from build123d import *

# Parameters (mm, degrees)
F1_DEPTH = 2


with BuildPart() as f1:
    # F0 (on Top) → F1 (new body)
    with BuildSketch(Plane.XY):
        with BuildLine():
            Line((-167, 135.5), (-167, 137.5))
            Line((-167, 137.5), (-169, 137.5))
            Line((-169, 137.5), (-172, 137.5))
            Line((-172, 137.5), (-172, 0))
            Line((-172, 0), (-170, 0))
            Line((-170, 0), (-170, 2))
            ThreePointArc((-170, 2), (-169.853553, 2.353553), (-169.5, 2.5))
            Line((-169.5, 2.5), (-167, 2.5))
            Line((-167, 2.5), (-167, 3.5))
            Line((-167, 3.5), (-167, 5.5))
            Line((-167, 5.5), (-167, 6.5))
            Line((-167, 6.5), (-169.5, 6.5))
            ThreePointArc((-169.5, 6.5), (-169.853553, 6.646447), (-170, 7))
            Line((-170, 7), (-170, 15))
            ThreePointArc((-170, 15), (-169.853553, 15.353553), (-169.5, 15.5))
            Line((-169.5, 15.5), (-167, 15.5))
            Line((-167, 15.5), (-167, 16.5))
            Line((-167, 16.5), (-167, 18.5))
            Line((-167, 18.5), (-167, 19.5))
            Line((-167, 19.5), (-169.5, 19.5))
            ThreePointArc((-169.5, 19.5), (-169.853553, 19.646447), (-170, 20))
            Line((-170, 20), (-170, 28))
            ThreePointArc((-170, 28), (-169.853553, 28.353553), (-169.5, 28.5))
            Line((-169.5, 28.5), (-167, 28.5))
            Line((-167, 28.5), (-167, 29.5))
            Line((-167, 29.5), (-167, 31.5))
            Line((-167, 31.5), (-167, 32.5))
            Line((-167, 32.5), (-169.5, 32.5))
            ThreePointArc((-169.5, 32.5), (-169.853553, 32.646447), (-170, 33))
            Line((-170, 33), (-170, 41))
            ThreePointArc((-170, 41), (-169.853553, 41.353553), (-169.5, 41.5))
            Line((-169.5, 41.5), (-167, 41.5))
            Line((-167, 41.5), (-167, 42.5))
            Line((-167, 42.5), (-167, 44.5))
            Line((-167, 44.5), (-167, 45.5))
            Line((-167, 45.5), (-169.5, 45.5))
            ThreePointArc((-169.5, 45.5), (-169.853553, 45.646447), (-170, 46))
            Line((-170, 46), (-170, 54))
            ThreePointArc((-170, 54), (-169.853553, 54.353553), (-169.5, 54.5))
            Line((-169.5, 54.5), (-167, 54.5))
            Line((-167, 54.5), (-167, 55.5))
            Line((-167, 55.5), (-167, 57.5))
            Line((-167, 57.5), (-167, 58.5))
            Line((-167, 58.5), (-169.5, 58.5))
            ThreePointArc((-169.5, 58.5), (-169.853553, 58.646447), (-170, 59))
            Line((-170, 59), (-170, 67))
            ThreePointArc((-170, 67), (-169.853553, 67.353553), (-169.5, 67.5))
            Line((-169.5, 67.5), (-167, 67.5))
            Line((-167, 67.5), (-167, 68.5))
            Line((-167, 68.5), (-167, 70.5))
            Line((-167, 70.5), (-167, 71.5))
            Line((-167, 71.5), (-169.5, 71.5))
            ThreePointArc((-169.5, 71.5), (-169.853553, 71.646447), (-170, 72))
            Line((-170, 72), (-170, 80))
            ThreePointArc((-170, 80), (-169.853553, 80.353553), (-169.5, 80.5))
            Line((-169.5, 80.5), (-167, 80.5))
            Line((-167, 80.5), (-167, 81.5))
            Line((-167, 81.5), (-167, 83.5))
            Line((-167, 83.5), (-167, 84.5))
            Line((-167, 84.5), (-169.5, 84.5))
            ThreePointArc((-169.5, 84.5), (-169.853553, 84.646447), (-170, 85))
            Line((-170, 85), (-170, 93))
            ThreePointArc((-170, 93), (-169.853553, 93.353553), (-169.5, 93.5))
            Line((-169.5, 93.5), (-167, 93.5))
            Line((-167, 93.5), (-167, 94.5))
            Line((-167, 94.5), (-167, 96.5))
            Line((-167, 96.5), (-167, 97.5))
            Line((-167, 97.5), (-169.5, 97.5))
            ThreePointArc((-169.5, 97.5), (-169.853553, 97.646447), (-170, 98))
            Line((-170, 98), (-170, 106))
            ThreePointArc((-170, 106), (-169.853553, 106.353553), (-169.5, 106.5))
            Line((-169.5, 106.5), (-167, 106.5))
            Line((-167, 106.5), (-167, 107.5))
            Line((-167, 107.5), (-167, 109.5))
            Line((-167, 109.5), (-167, 110.5))
            Line((-167, 110.5), (-169.5, 110.5))
            ThreePointArc((-169.5, 110.5), (-169.853553, 110.646447), (-170, 111))
            Line((-170, 111), (-170, 119))
            ThreePointArc((-170, 119), (-169.853553, 119.353553), (-169.5, 119.5))
            Line((-169.5, 119.5), (-167, 119.5))
            Line((-167, 119.5), (-167, 120.5))
            Line((-167, 120.5), (-167, 122.5))
            Line((-167, 122.5), (-167, 123.5))
            Line((-167, 123.5), (-169.5, 123.5))
            ThreePointArc((-169.5, 123.5), (-169.853553, 123.646447), (-170, 124))
            Line((-170, 124), (-170, 132))
            ThreePointArc((-170, 132), (-169.853553, 132.353553), (-169.5, 132.5))
            Line((-169.5, 132.5), (-167, 132.5))
            Line((-167, 132.5), (-167, 133.5))
            Line((-167, 133.5), (-167, 135.5))
        make_face()
        Polygon((-167, 5.5), (-167, 3.5), (-165.5, 3.5), (-165.5, 3), (-165, 3.5), (-165, 5.5), (-165.5, 6), (-165.5, 5.5), align=None)
        Polygon((-167, 18.5), (-167, 16.5), (-165.5, 16.5), (-165.5, 16), (-165, 16.5), (-165, 18.5), (-165.5, 19), (-165.5, 18.5), align=None)
        Polygon((-167, 31.5), (-167, 29.5), (-165.5, 29.5), (-165.5, 29), (-165, 29.5), (-165, 31.5), (-165.5, 32), (-165.5, 31.5), align=None)
        Polygon((-167, 44.5), (-167, 42.5), (-165.5, 42.5), (-165.5, 42), (-165, 42.5), (-165, 44.5), (-165.5, 45), (-165.5, 44.5), align=None)
        Polygon((-167, 57.5), (-167, 55.5), (-165.5, 55.5), (-165.5, 55), (-165, 55.5), (-165, 57.5), (-165.5, 58), (-165.5, 57.5), align=None)
        Polygon((-165.5, 70.5), (-167, 70.5), (-167, 68.5), (-165.5, 68.5), (-165.5, 68), (-165, 68.5), (-165, 70.5), (-165.5, 71), align=None)
        Polygon((-165.5, 83.5), (-167, 83.5), (-167, 81.5), (-165.5, 81.5), (-165.5, 81), (-165, 81.5), (-165, 83.5), (-165.5, 84), align=None)
        Polygon((-165.5, 96.5), (-167, 96.5), (-167, 94.5), (-165.5, 94.5), (-165.5, 94), (-165, 94.5), (-165, 96.5), (-165.5, 97), align=None)
        Polygon((-165.5, 109.5), (-167, 109.5), (-167, 107.5), (-165.5, 107.5), (-165.5, 107), (-165, 107.5), (-165, 109.5), (-165.5, 110), align=None)
        Polygon((-165.5, 122.5), (-167, 122.5), (-167, 120.5), (-165.5, 120.5), (-165.5, 120), (-165, 120.5), (-165, 122.5), (-165.5, 123), align=None)
        Polygon((-165.5, 135.5), (-167, 135.5), (-167, 133.5), (-165.5, 133.5), (-165.5, 133), (-165, 133.5), (-165, 135.5), (-165.5, 136), align=None)
        with BuildLine():
            Line((-169, 137.5), (-167, 137.5))
            Line((-167, 137.5), (-167, 145))
            ThreePointArc((-167, 145), (-167.146447, 145.353553), (-167.5, 145.5))
            Line((-167.5, 145.5), (-168.5, 145.5))
            ThreePointArc((-168.5, 145.5), (-168.853553, 145.353553), (-169, 145))
            Line((-169, 145), (-169, 137.5))
        make_face()
    extrude(amount=F1_DEPTH)


solid = f1.part
CAD build for the part. Positions are in the model's coordinates, mm. Give positions to 0.01 mm unless a question says otherwise; leave off trailing zeros. Write each loop counter-clockwise with the first axis right and the second up, starting at its lowest first coordinate (ties: lowest second). Pieces come first, ordered by that corner, then holes. Notation, with made-up numbers: M 40,-36.75 L 57,-36.75 A30 ccw 57,-6.75 Z; hole C -10.5,54 d3. An arc over 180 degrees is marked long. Put each result on its own line as item: value. Start each with the question number.
(1) Probe L1, parallel to X at y = 74, z = 0.5; L2, parallel to X at y = 139, z = 0.95; L3, parallel to Y at x = -171.5, z = 0.9. List the from-to ranges inside material, lowest first.
(2) Flat gauge pins, fed straight in: pin 1 Ø0.5 at (y, z) = (29, 1.5) entering from +X; pin 2 Ø0.6 at (y, z) = (22.5, 1) entering from +X; pin 3 Ø1 at (x, z) = (-167.5, 1) entering from -Y. Where does each tip first touch, or does it go through?
(3) Band-saw the part on A-A, the plane y = 51.5. Write the cut outline in (x, z), and give its area (3 significant figures).
Response values:
1. L1: x = -172 to -170
1. L2: x = -169 to -167
1. L3: y = 0 to 137.5
2. pin 1: stops at x = -165.25
2. pin 2: stops at x = -170
2. pin 3: stops at y = 2.5
3. outline: M -172,0 L -170,0 L -170,2 L -172,2 Z
3. area: 4.00 mm2
